```python
from build123d import *

# Parameters (mm, degrees)
SKETCH1_W               = 90
SKETCH1_H               = 46
SKETCH1_R               = 2
BOSS_EXTRUDE1_DEPTH     = 6.35
M2_CLEARANCE_HOLE1_D    = 2.2
CUT_EXTRUDE1_DEPTH      = 7.35
CUT_EXTRUDE2_DEPTH      = 7.35
SKETCH8_W               = 25
SKETCH8_H               = 6.35
BOSS_EXTRUDE2_DEPTH     = 10
FILLET1_R               = 3
MIRROR5_COPY_1_SKETCH_W = 90
MIRROR5_COPY_1_SKETCH_H = 46
MIRROR5_COPY_1_SKETCH_R = 2
MIRROR5_COPY_1_DEPTH    = 6.35
MIRROR5_COPY_2_D        = 2.2
MIRROR5_COPY_3_DEPTH    = 7.35
MIRROR5_COPY_4_DEPTH    = 7.35
MIRROR5_COPY_5_D        = 2.2
MIRROR5_COPY_6_DEPTH    = 7.35
MIRROR5_COPY_7_DEPTH    = 7.35
FILLET1_OF_MIRROR5_R    = 3
SKETCH9_R               = 2
CUT_EXTRUDE3_DEPTH      = 10
SKETCH10_R              = 2
CUT_EXTRUDE4_DEPTH      = 6.35
SKETCH12_R              = 1.5
CUT_EXTRUDE6_DEPTH      = 7.35
SKETCH11_W              = 52
SKETCH11_H              = 3
CUT_EXTRUDE7_DEPTH      = 2


with BuildPart() as part:
    # Sketch1 → Boss-Extrude1 (new body)
    with BuildSketch(Plane(origin=(0, 0, 0), x_dir=(1, 0, 0), z_dir=(0, 1, 0))):
        with Locations((45, 23)):
            Rectangle(SKETCH1_W, SKETCH1_H)
        with Locations((45, 5)):
            Circle(SKETCH1_R, mode=Mode.SUBTRACT)
        with Locations((5, 23)):
            Circle(SKETCH1_R, mode=Mode.SUBTRACT)
        with Locations((85, 23)):
            Circle(SKETCH1_R, mode=Mode.SUBTRACT)
    boss_extrude1 = extrude(amount=BOSS_EXTRUDE1_DEPTH)

    # M2 Clearance Hole1 (through all)
    with Locations(Plane(origin=(0, 6.35, 0), x_dir=(1, 0, 0), z_dir=(0, 1, 0))):
        with Locations((13.5, 26), (13.5, 20), (24, 25.5), (24, 20.5), (38, 25.5), (38, 20.5), (52, 25.5), (52, 20.5), (66, 25.5), (66, 20.5), (76.5, 26), (76.5, 20)):
            m2_clearance_hole1 = Hole(M2_CLEARANCE_HOLE1_D / 2)

    # Sketch6 → Cut-Extrude1 (cut, through all)
    with BuildSketch(Plane(origin=(0, 6.35, 0), x_dir=(1, 0, 0), z_dir=(0, 1, 0))):
        with BuildLine():
            Line((18, 28), (18, 18))
            ThreePointArc((18, 18), (17.25, 17.25), (16.5, 18))
            Line((16.5, 18), (16.5, 28))
            ThreePointArc((16.5, 28), (17.25, 28.75), (18, 28))
        make_face()
    cut_extrude1 = extrude(amount=-CUT_EXTRUDE1_DEPTH, mode=Mode.SUBTRACT)

    # Sketch7 → Cut-Extrude2 (cut, through all)
    with BuildSketch(Plane(origin=(0, 6.35, 0), x_dir=(1, 0, 0), z_dir=(0, 1, 0))):
        with BuildLine():
            Line((31.5, 28), (31.5, 18))
            ThreePointArc((31.5, 18), (30.75, 17.25), (30, 18))
            Line((30, 18), (30, 28))
            ThreePointArc((30, 28), (30.75, 28.75), (31.5, 28))
        make_face()
        with BuildLine():
            Line((44, 28), (44, 18))
            ThreePointArc((44, 18), (44.75, 17.25), (45.5, 18))
            Line((45.5, 18), (45.5, 28))
            ThreePointArc((45.5, 28), (44.75, 28.75), (44, 28))
        make_face()
        with BuildLine():
            Line((58, 28), (58, 18))
            ThreePointArc((58, 18), (58.75, 17.25), (59.5, 18))
            Line((59.5, 18), (59.5, 28))
            ThreePointArc((59.5, 28), (58.75, 28.75), (58, 28))
        make_face()
        with BuildLine():
            Line((73.5, 28), (73.5, 18))
            ThreePointArc((73.5, 18), (72.75, 17.25), (72, 18))
            Line((72, 18), (72, 28))
            ThreePointArc((72, 28), (72.75, 28.75), (73.5, 28))
        make_face()
    cut_extrude2 = extrude(amount=-CUT_EXTRUDE2_DEPTH, mode=Mode.SUBTRACT)

    # Mirror1: Boss-Extrude1, M2 Clearance Hole1, Cut-Extrude1, Cut-Extrude2 across plane
    add(boss_extrude1.mirror(Plane(origin=(0, 0, -46), x_dir=(1, 0, 0), z_dir=(0, 0, -1))))
    add(m2_clearance_hole1.mirror(Plane(origin=(0, 0, -46), x_dir=(1, 0, 0), z_dir=(0, 0, -1))), mode=Mode.SUBTRACT)
    add(cut_extrude1.mirror(Plane(origin=(0, 0, -46), x_dir=(1, 0, 0), z_dir=(0, 0, -1))), mode=Mode.SUBTRACT)
    add(cut_extrude2.mirror(Plane(origin=(0, 0, -46), x_dir=(1, 0, 0), z_dir=(0, 0, -1))), mode=Mode.SUBTRACT)

    # Sketch8 → Boss-Extrude2 (add)
    with BuildSketch(Plane(origin=(90, 0, 0), x_dir=(0, 0, -1), z_dir=(1, 0, 0))):
        with Locations((12.5, 3.175)):
            Rectangle(SKETCH8_W, SKETCH8_H)
        with Locations((79.5, 3.175)):
            Rectangle(SKETCH8_W, SKETCH8_H)
    boss_extrude2 = extrude(amount=BOSS_EXTRUDE2_DEPTH)

    # Fillet1
    fillet1_edges = [part.edges().sort_by_distance(p)[0] for p in [
        (100, 3.175, 0),
        (100, 3.175, -25),
        (100, 3.175, -92),
        (100, 3.175, -67),
    ]]
    fillet(fillet1_edges, radius=FILLET1_R)

    # Mirror5: Boss-Extrude1, Boss-Extrude2 across plane
    add(boss_extrude1.mirror(Plane.ZY.offset(-45)))
    add(boss_extrude2.mirror(Plane.ZY.offset(-45)))

    # Mirror5 copy 1 sketch → Mirror5 copy 1 (add)
    with BuildSketch(Plane(origin=(90, 0, -92), x_dir=(-1, 0, 0), z_dir=(0, 1, 0))):
        with Locations((45, 23)):
            Rectangle(MIRROR5_COPY_1_SKETCH_W, MIRROR5_COPY_1_SKETCH_H)
        with Locations((45, 5)):
            Circle(MIRROR5_COPY_1_SKETCH_R, mode=Mode.SUBTRACT)
        with Locations((5, 23)):
            Circle(MIRROR5_COPY_1_SKETCH_R, mode=Mode.SUBTRACT)
        with Locations((85, 23)):
            Circle(MIRROR5_COPY_1_SKETCH_R, mode=Mode.SUBTRACT)
    extrude(amount=MIRROR5_COPY_1_DEPTH)

    # Mirror5 copy 2 (through all)
    with Locations(Plane(origin=(90, 6.35, -92), x_dir=(-1, 0, 0), z_dir=(0, 1, 0))):
        with Locations((13.5, 26), (13.5, 20), (24, 25.5), (24, 20.5), (38, 25.5), (38, 20.5), (52, 25.5), (52, 20.5), (66, 25.5), (66, 20.5), (76.5, 26), (76.5, 20)):
            Hole(MIRROR5_COPY_2_D / 2)

    # Mirror5 copy 3 sketch → Mirror5 copy 3 (cut, through all)
    with BuildSketch(Plane(origin=(90, 6.35, -92), x_dir=(-1, 0, 0), z_dir=(0, 1, 0))):
        with BuildLine():
            Line((18, 28), (18, 18))
            ThreePointArc((18, 18), (17.25, 17.25), (16.5, 18))
            Line((16.5, 18), (16.5, 28))
            ThreePointArc((16.5, 28), (17.25, 28.75), (18, 28))
        make_face()
    extrude(amount=-MIRROR5_COPY_3_DEPTH, mode=Mode.SUBTRACT)

    # Mirror5 copy 4 sketch → Mirror5 copy 4 (cut, through all)
    with BuildSketch(Plane(origin=(90, 6.35, -92), x_dir=(-1, 0, 0), z_dir=(0, 1, 0))):
        with BuildLine():
            Line((31.5, 28), (31.5, 18))
            ThreePointArc((31.5, 18), (30.75, 17.25), (30, 18))
            Line((30, 18), (30, 28))
            ThreePointArc((30, 28), (30.75, 28.75), (31.5, 28))
        make_face()
        with BuildLine():
            Line((44, 28), (44, 18))
            ThreePointArc((44, 18), (44.75, 17.25), (45.5, 18))
            Line((45.5, 18), (45.5, 28))
            ThreePointArc((45.5, 28), (44.75, 28.75), (44, 28))
        make_face()
        with BuildLine():
            Line((58, 28), (58, 18))
            ThreePointArc((58, 18), (58.75, 17.25), (59.5, 18))
            Line((59.5, 18), (59.5, 28))
            ThreePointArc((59.5, 28), (58.75, 28.75), (58, 28))
        make_face()
        with BuildLine():
            Line((73.5, 28), (73.5, 18))
            ThreePointArc((73.5, 18), (72.75, 17.25), (72, 18))
            Line((72, 18), (72, 28))
            ThreePointArc((72, 28), (72.75, 28.75), (73.5, 28))
        make_face()
    extrude(amount=-MIRROR5_COPY_4_DEPTH, mode=Mode.SUBTRACT)

    # Mirror5 copy 5 (through all)
    with Locations(Plane(origin=(90, 6.35, 0), x_dir=(-1, 0, 0), z_dir=(0, 1, 0))):
        with Locations((13.5, -26), (13.5, -20), (24, -25.5), (24, -20.5), (38, -25.5), (38, -20.5), (52, -25.5), (52, -20.5), (66, -25.5), (66, -20.5), (76.5, -26), (76.5, -20)):
            Hole(MIRROR5_COPY_5_D / 2)

    # Mirror5 copy 6 sketch → Mirror5 copy 6 (cut, through all)
    with BuildSketch(Plane(origin=(90, 6.35, 0), x_dir=(-1, 0, 0), z_dir=(0, 1, 0))):
        with BuildLine():
            Line((18, -28), (18, -18))
            ThreePointArc((18, -18), (17.25, -17.25), (16.5, -18))
            Line((16.5, -18), (16.5, -28))
            ThreePointArc((16.5, -28), (17.25, -28.75), (18, -28))
        make_face()
    extrude(amount=-MIRROR5_COPY_6_DEPTH, mode=Mode.SUBTRACT)

    # Mirror5 copy 7 sketch → Mirror5 copy 7 (cut, through all)
    with BuildSketch(Plane(origin=(90, 6.35, 0), x_dir=(-1, 0, 0), z_dir=(0, 1, 0))):
        with BuildLine():
            Line((31.5, -28), (31.5, -18))
            ThreePointArc((31.5, -18), (30.75, -17.25), (30, -18))
            Line((30, -18), (30, -28))
            ThreePointArc((30, -28), (30.75, -28.75), (31.5, -28))
        make_face()
        with BuildLine():
            Line((44, -28), (44, -18))
            ThreePointArc((44, -18), (44.75, -17.25), (45.5, -18))
            Line((45.5, -18), (45.5, -28))
            ThreePointArc((45.5, -28), (44.75, -28.75), (44, -28))
        make_face()
        with BuildLine():
            Line((58, -28), (58, -18))
            ThreePointArc((58, -18), (58.75, -17.25), (59.5, -18))
            Line((59.5, -18), (59.5, -28))
            ThreePointArc((59.5, -28), (58.75, -28.75), (58, -28))
        make_face()
        with BuildLine():
            Line((73.5, -28), (73.5, -18))
            ThreePointArc((73.5, -18), (72.75, -17.25), (72, -18))
            Line((72, -18), (72, -28))
            ThreePointArc((72, -28), (72.75, -28.75), (73.5, -28))
        make_face()
    extrude(amount=-MIRROR5_COPY_7_DEPTH, mode=Mode.SUBTRACT)

    # Fillet1 of Mirror5
    fillet1_of_mirror5_edges = [part.edges().sort_by_distance(p)[0] for p in [
        (-10, 3.175, 0),
        (-10, 3.175, -25),
        (-10, 3.175, -92),
        (-10, 3.175, -67),
    ]]
    fillet(fillet1_of_mirror5_edges, radius=FILLET1_OF_MIRROR5_R)

    # Sketch9 → Cut-Extrude3 (cut)
    with BuildSketch(Plane(origin=(0, 6.35, 0), x_dir=(1, 0, 0), z_dir=(0, 1, 0))):
        with Locations((5, 5)):
            Circle(SKETCH9_R)
        with Locations((85, 5)):
            Circle(SKETCH9_R)
        with Locations((85, 87)):
            Circle(SKETCH9_R)
        with Locations((5, 87)):
            Circle(SKETCH9_R)
    extrude(amount=-CUT_EXTRUDE3_DEPTH, mode=Mode.SUBTRACT)

    # Sketch10 → Cut-Extrude4 (cut)
    with BuildSketch(Plane.XZ):
        with Locations((85, -46)):
            Circle(SKETCH10_R)
        with Locations((45, -46)):
            Circle(SKETCH10_R)
        with Locations((5, -46)):
            Circle(SKETCH10_R)
    extrude(amount=-CUT_EXTRUDE4_DEPTH, mode=Mode.SUBTRACT)

    # Sketch12 → Cut-Extrude6 (cut, through all)
    with BuildSketch(Plane(origin=(0, 6.35, 0), x_dir=(1, 0, 0), z_dir=(0, 1, 0))):
        with Locations((13.5, 12.75)):
            Circle(SKETCH12_R)
        with Locations((13.5, 33.25)):
            Circle(SKETCH12_R)
        with Locations((76.5, 33.25)):
            Circle(SKETCH12_R)
        with Locations((76.5, 12.75)):
            Circle(SKETCH12_R)
    cut_extrude6 = extrude(amount=-CUT_EXTRUDE6_DEPTH, mode=Mode.SUBTRACT)

    # Mirror7: Cut-Extrude6 across plane
    add(cut_extrude6.mirror(Plane(origin=(0, 0, -46), x_dir=(1, 0, 0), z_dir=(0, 0, -1))), mode=Mode.SUBTRACT)

    # Sketch11 → Cut-Extrude7 (cut)
    with BuildSketch(Plane(origin=(0, 6.35, 0), x_dir=(1, 0, 0), z_dir=(0, 1, 0))):
        with Locations((45, 12.75)):
            Rectangle(SKETCH11_W, SKETCH11_H)
        with Locations((45, 33.25)):
            Rectangle(SKETCH11_W, SKETCH11_H)
        with Locations((45, 58.75)):
            Rectangle(SKETCH11_W, SKETCH11_H)
        with Locations((45, 79.25)):
            Rectangle(SKETCH11_W, SKETCH11_H)
    extrude(amount=-CUT_EXTRUDE7_DEPTH, mode=Mode.SUBTRACT)


solid = part.part
```
For this review, take the finished solid that the model builds, in its own axes (mm). A direction names the side the tool comes from. Give positions to 0.01 mm unless a question says otherwise; leave off trailing zeros. Write each loop counter-clockwise with the first axis right and the second up, starting at its lowest first coordinate (ties: lowest second). Pieces come first, ordered by that corner, then holes. Notation, with made-up numbers: M 88.25,-19 L 103.25,-19 A22 ccw 103.25,-2 Z; hole C -38.5,73.25 d5. An arc over 180 degrees is marked long. Answer as a JSON object with one key per item and string values. Group by question number.
Item 1: For pin 1 Ø1.3 at (x, z) = (66, -25.5) entering from -Y; pin 2 Ø1.9 at (y, z) = (2, -25) entering from -X, all flat-tipped, find the tip position at first contact; note any pin that passes through.
Item 2: For probe 1 along X at (y, z) = (4.25, -58.75); probe 2 along Z at (x, y) = (91, 2.5); probe 3 along X at (y, z) = (2, -5.5), list the stretches that pass through material, from the lowest coordinate up. Write a range as [from, to].
Item 3: Consider section A-A on z = -33.25. Write out the cut boundary in (x, y).
Item 4: Tool access review of faces 5 (the flat face through (72, 3, -69)), 6 (the flat face through (90, 3, -46)), 7 (the cylindrical face through (-9.14, 3.22, -67.9)): name each direction out of +Z, -Z, +X, -X, +Y, -Y from which nothing blocks a thin tool from reaching the whole face with its end or side.
Item 5: Consider section D-D on y = 1.75. Count the separate pieces of the cut face and the enclosed holes in it, plus the area to 3 significant figures.
Item 6: Draft analysis for pull direction X (two halves, no side actions). For faces 1 (the flat face through (58.5, 3, -23)), 2 (the cylindrical face through (99.1, 3.22, -0.86)), 3 (the cylindrical face through (38.59, 3.13, -70.57)), 4 (the cylindrical face through (-9.14, 3.22, -24.1)), state which applies: +X half, -X half, draft (parallel to the pull), parting line (faces both ways), or undercut.
Item 7: Consider section C-C on z = -12.75. Write out the cut boundary in (x, y).
Item 8: Consider section B-B on x = 5. Write out the cut boundary in (y, z).
Check result:
{
 "1": {"pin 1": "passes through", "pin 2": "stops at x = -9.19"},
 "2": {"probe 1": "x = [0, 12], [15, 75], [78, 90]", "probe 2": "z = [-92, -67], [-25, 0]", "probe 3": "x = [-10, 3.06], [6.94, 43.06], [46.94, 83.06], [86.94, 100]"},
 "3": {"outline": "M 0,0 L 12,0 L 12,6.35 L 0,6.35 Z; M 15,0 L 75,0 L 75,6.35 L 71,6.35 L 71,4.35 L 19,4.35 L 19,6.35 L 15,6.35 Z; M 78,0 L 90,0 L 90,6.35 L 78,6.35 Z"},
 "4": {"face 5": "+Y, -Y", "face 6": "+X, +Y, -Y", "face 7": "-X, +Y, -Y"},
 "5": {"separate pieces": "1", "enclosed holes": "55", "area": "8,790 mm^2"},
 "6": {"face 1": "undercut", "face 2": "+X half", "face 3": "undercut", "face 4": "-X half"},
 "7": {"outline": "M -10,0 L 12,0 L 12,6.35 L -10,6.35 Z; M 15,0 L 75,0 L 75,6.35 L 71,6.35 L 71,4.35 L 19,4.35 L 19,6.35 L 15,6.35 Z; M 78,0 L 100,0 L 100,6.35 L 78,6.35 Z"},
 "8": {"outline": "M 0,-92 L 6.35,-92 L 6.35,-89 L 0,-89 Z; M 0,-85 L 6.35,-85 L 6.35,-71 L 0,-71 Z; M 0,-67 L 6.35,-67 L 6.35,-48 L 0,-48 Z; M 0,-44 L 6.35,-44 L 6.35,-25 L 0,-25 Z; M 0,-21 L 6.35,-21 L 6.35,-7 L 0,-7 Z; M 0,-3 L 6.35,-3 L 6.35,0 L 0,0 Z"}
}
